Part print with two shaded views. Sizes in mm from the minimum x, y, z corner. Round coordinates to 2 decimals unless told otherwise and drop trailing zeros. Order: outer loops, then holes, each group sorted by start corner. A loop starts at its lowest first (then second) coordinate and runs counter-clockwise, first axis right, second up. Notation, with made-up numbers: (53, -18.5) - (91, -18.5) arc R30 ccw to (91, 7.5) - close; hole circle Ø8 at (65.5, -12). An arc over 180 degrees is marked (long way). Answer as CSV lines item,"result". Start each with the question number.
1. Band-saw the part on C-C on y = 2.05. List the corners of the cut face in (x, z) (3 decimals), then the cut area to 3 significant figures.
2. Band-saw the part on B-B on x = 9. List the corners of the cut face in (y, z) (3 decimals).
3. Band-saw the part on A-A on z = 40.5. List the corners of the cut face in (x, y) (3 decimals), then the cut area to 3 significant figures.
4. Wall check: line 1 along Z through (x, y) = (18, 1.4); line 2 along X through (y, z) = (0.15, 40) (3 decimals); line 3 along Z through (x, y) = (14.5, 2.4). Give the ranges that are in metal, low to high. Write a range as [from, to].
5. Pin check, flat tip, straight feed: pin 1 Ø2 at (x, z) = (26, 55.5) entering from -Y. Stop position of the tip, or through.
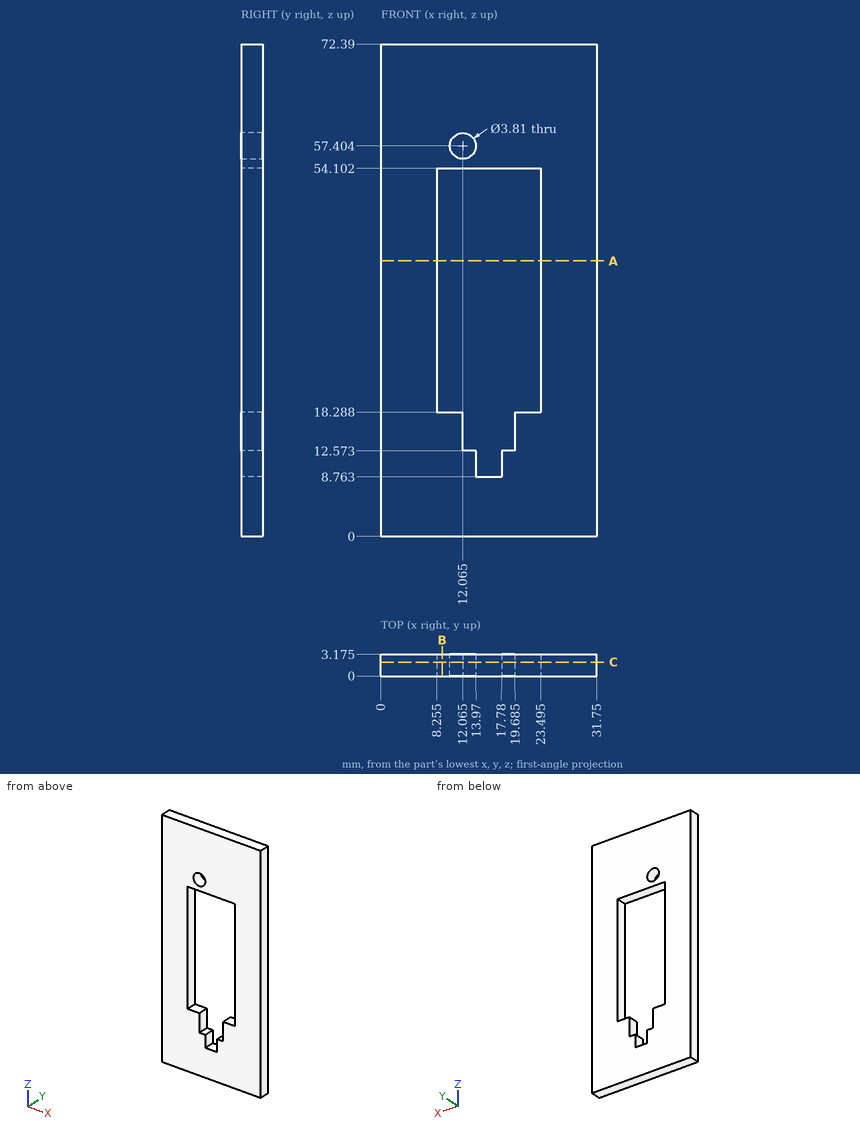
Reply:
1,outline,"(0, 0) - (31.75, 0) - (31.75, 72.39) - (0, 72.39) - close; hole (8.255, 18.288) - (12.065, 18.288) - (12.065, 12.573) - (13.97, 12.573) - (13.97, 8.763) - (17.78, 8.763) - (17.78, 12.573) - (19.685, 12.573) - (19.685, 18.288) - (23.495, 18.288) - (23.495, 54.102) - (8.255, 54.102) - close; hole circle Ø3.81 at (12.065, 57.404)"
1,area,"1,680 mm2"
2,outline,"(0, 0) - (3.175, 0) - (3.175, 18.288) - (0, 18.288) - close; (0, 54.102) - (3.175, 54.102) - (3.175, 72.39) - (0, 72.39) - close"
3,outline,"(0, 0) - (8.255, 0) - (8.255, 3.175) - (0, 3.175) - close; (23.495, 0) - (31.75, 0) - (31.75, 3.175) - (23.495, 3.175) - close"
3,area,"52.4 mm2"
4,line 1,"z = [0, 12.57], [54.1, 72.39]"
4,line 2,"x = [0, 8.255], [23.495, 31.75]"
4,line 3,"z = [0, 8.76], [54.1, 72.39]"
5,pin 1,"stops at y = 0"
